Design review of the part built by this model. Coordinates are the model's own, in mm. Face numbers are marked on the shaded views. A direction names the side the tool comes from. Give positions to 0.01 mm unless a question says otherwise; leave off trailing zeros. Order: outer loops, then holes, each group sorted by start corner. A loop starts at its lowest first (then second) coordinate and runs counter-clockwise, first axis right, second up. Notation, with made-up numbers: (58, 87.5) -> (92, 87.5) arc R20 ccw to (92, 117.5) -> close; hole circle Ø6 at (5, 43). An arc over 180 degrees is marked (long way). One line per item, written item: value. Start each with the question number.
1) The part is to be moulded in two halves that separate along X. For the marked faces 1, 2, 3 and 4, say which applies: released by +X, released by -X, zero draft, split by the parting line, or undercut.
2) Consider section A-A (x = 38.1). State the section outline as (y, z) points, plus the area to 3 significant figures.
3) Consider section C-C (y = 74). State the section outline as (x, z) points.
4) For pin 1 (21 mm diameter, centred on x = 44.5, z = -11.5, fed in from -Y); pin 2 (8 mm diameter, centred on x = 45.5, y = 74.5, fed in from +Z), all flat-tipped, find the tip position at first contact; note any pin that passes through.
5) Tool access review of the marked faces 5, 6 and 7: name each direction out of +Z, -Z, +X, -X, +Y, -Y from which nothing blocks a thin tool from reaching the whole face with its end or side.
6) Consider section B-B (z = -3.5). State the section outline as (x, y) points (3 decimals).
7) Wall thickness on line 1 along Y through (x, z) = (38, -9); line 2 along Y through (x, z) = (53, 40); line 3 along X through (y, z) = (75.5, -12): over which ranges is each line inside the solid? List them lowest first. Write a range as from..to.
8) Consider section D-D (z = 17). State the section outline as (x, y) points.
Autodesk Inventor part; units mm, degrees
ref_plane "YZ Plane" through (0, 0, 0) normal (1, 0, 0) x (0, 1, 0)
ref_plane "XZ Plane" through (0, 0, 0) normal (0, 1, 0) x (-1, 0, 0)
ref_plane "XY Plane" through (0, 0, 0) normal (0, 0, 1) x (1, 0, 0)
sketch "Sketch1" plane through (0, 0, 0) normal (0, 0, 1) x (1, 0, 0)
  line L0 (0, 0) -> (12.7, 0)
  line L1 (12.7, 0) -> (12.7, 38.1)
  line L2 (12.7, 38.1) -> (63.5, 38.1)
  line L3 (63.5, 38.1) -> (63.5, 0)
  line L4 (63.5, 0) -> (76.2, 0)
  line L5 (76.2, 0) -> (76.2, 114.3)
  line L6 (76.2, 114.3) -> (0, 114.3)
  line L7 (0, 114.3) -> (0, 0)
  circle A0 centre (38.1, 67.818) radius 9.525
  dimension "d0" = 12.7
  dimension "d1" = 50.8
  dimension "d2" = 76.2
  dimension "d3" = 114.3
  dimension "d4" = 38.1
  dimension "d5" = 19.05
  dimension "d6" = 67.818
  dimension "d7" = 38.1
extrude "Extrusion1" add sketch "Sketch1" against normal blind 19.05
sketch "Sketch3" plane through (0, 114.3, 0) normal (0, 1, 0) x (1, 0, 0)
  line L0 (0, 0) -> (0, -38.1)
  line L1 (0, -38.1) -> (25.4, -63.5)
  line L2 (25.4, -63.5) -> (76.2, -63.5)
  line L3 (0, 0) -> (12.7, 0)
  line L4 (76.2, -63.5) -> (76.2, 0)
  line L5 (76.2, 0) -> (0, 0)
  dimension "d10" = 90
  dimension "d11" = 90
  dimension "d12" = 50.8
  dimension "d13" = 25.4
  dimension "d14" = 63.5
extrude "Extrusion2" add sketch "Sketch3" against normal blind 19.05
properties part number "HW 2 Part 6"
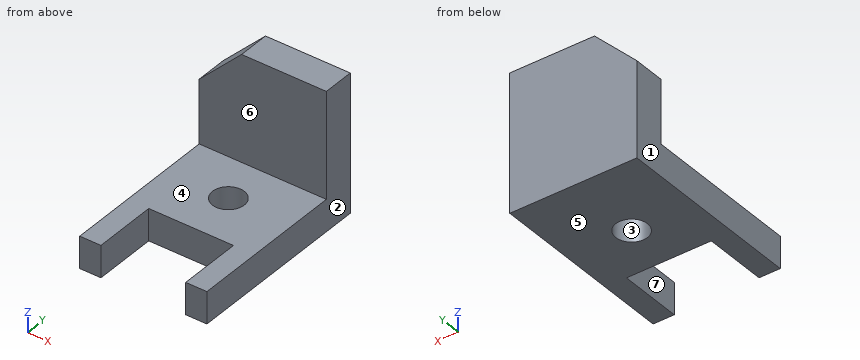
Checked values:
1. face 1: released by -X
1. face 2: released by +X
1. face 3: undercut
1. face 4: zero draft
2. outline: (38.1, -19.05) -> (58.29, -19.05) -> (58.29, 0) -> (38.1, 0) -> close; (77.34, -19.05) -> (114.3, -19.05) -> (114.3, 63.5) -> (95.25, 63.5) -> (95.25, 0) -> (77.34, 0) -> close
2. area: 2,300 mm^2
3. outline: (0, -19.05) -> (30.85, -19.05) -> (30.85, 0) -> (0, 0) -> close; (45.35, -19.05) -> (76.2, -19.05) -> (76.2, 0) -> (45.35, 0) -> close
4. pin 1: stops at y = 38.1
4. pin 2: stops at z = 0
5. face 5: -Z, +X, -X, +Y, -Y
5. face 6: +Z, +X, -X, -Y
5. face 7: +Z, -Z, -Y
6. outline: (0, 0) -> (12.7, 0) -> (12.7, 38.1) -> (63.5, 38.1) -> (63.5, 0) -> (76.2, 0) -> (76.2, 114.3) -> (0, 114.3) -> close; hole circle Ø19.05 at (38.1, 67.818)
7. line 1: y = 38.1..58.29, 77.34..114.3
7. line 2: y = 95.25..114.3
7. line 3: x = 0..32.47, 43.73..76.2
8. outline: (0, 95.25) -> (76.2, 95.25) -> (76.2, 114.3) -> (0, 114.3) -> close
